```python
from build123d import *

# Parameters (mm, degrees)
F1_DEPTH    = 50.8
F2_R        = 1.75
F3_DEPTH    = 25.4
F5_T4_DEPTH = 50.8
F5_S5_R     = 1.75
F5_T6_DEPTH = 27
F5_S7_R     = 1.75
F5_T8_DEPTH = 27
F2_R_2      = 3
F6_DEPTH    = 7.511
F7_DEPTH    = 2.54
F4_R        = 1.75
F8_DEPTH    = 2.54


# Not quite as in the source:
# - a fillet or chamfer that OpenCascade refuses, or shapes differently, is made with other operations: its cross-section is extruded or revolved along the edge and cut away or added


with BuildPart() as f1:
    # F0 (on Top) → F1 (new body)
    with BuildSketch(Plane.XY):
        Polygon((0, 17.78), (0, 0), (17.78, 0), (17.78, 2.54), (2.54, 2.54), (2.54, 17.78), align=None)
    extrude(amount=F1_DEPTH)

    # F2 (on face) → F3 (cut)
    with BuildSketch(Plane(origin=(0, 0, 0), x_dir=(0, -1, 0), z_dir=(-1, 0, 0))):
        with Locations((-5.65, 9.9)):
            Circle(F2_R)
        with Locations((-5.65, 40.9)):
            Circle(F2_R)
    extrude(amount=-F3_DEPTH, mode=Mode.SUBTRACT)

    # F5: chamfer of 5.08 on 1 edges, made by hand


with BuildPart() as f5_tool2:
    # F5_s3 → F5_t4 (new body)
    with BuildSketch(Plane.XY):
        Polygon((2.54, 7.62), (7.62, 2.54), (2.54, 2.54), align=None)
    extrude(amount=F5_T4_DEPTH)

    # F5_s5 → F5_t6 (cut, symmetric)
    with BuildSketch(Plane.YZ.offset(5.1)):
        with Locations((5.65, 40.9)):
            Circle(F5_S5_R)
    extrude(amount=F5_T6_DEPTH, both=True, mode=Mode.SUBTRACT)

    # F5_s7 → F5_t8 (cut, symmetric)
    with BuildSketch(Plane.YZ.offset(5.1)):
        with Locations((5.65, 9.9)):
            Circle(F5_S7_R)
    extrude(amount=F5_T8_DEPTH, both=True, mode=Mode.SUBTRACT)


with BuildPart() as f1_1:
    add(f1.part)

    # F5_t1: union F5_tool2
    add(f5_tool2.part)

    # F2 (on face) → F6 (cut, through all)
    with BuildSketch(Plane(origin=(0, 0, 0), x_dir=(0, -1, 0), z_dir=(-1, 0, 0))):
        with Locations((-5.65, 40.9)):
            Circle(F2_R_2)
        with Locations((-5.65, 40.9)):
            Circle(F2_R, mode=Mode.SUBTRACT)
        with Locations((-5.65, 9.9)):
            Circle(F2_R_2)
        with Locations((-5.65, 9.9)):
            Circle(F2_R, mode=Mode.SUBTRACT)
    extrude(amount=-F6_DEPTH, mode=Mode.SUBTRACT)

    # F2 (on face) → F7 (join)
    with BuildSketch(Plane(origin=(0, 0, 0), x_dir=(0, -1, 0), z_dir=(-1, 0, 0))):
        with Locations((-5.65, 40.9)):
            Circle(F2_R_2)
        with Locations((-5.65, 40.9)):
            Circle(F2_R, mode=Mode.SUBTRACT)
        with Locations((-5.65, 9.9)):
            Circle(F2_R_2)
        with Locations((-5.65, 9.9)):
            Circle(F2_R, mode=Mode.SUBTRACT)
    extrude(amount=-F7_DEPTH)

    # F4 (on face) → F8 (cut, through all)
    with BuildSketch(Plane.XZ):
        with Locations((12.7, 45.72)):
            Circle(F4_R)
        with Locations((12.7, 5.08)):
            Circle(F4_R)
    extrude(amount=-F8_DEPTH, mode=Mode.SUBTRACT)


solid = f1_1.part
```
CAD build for the part. Positions are in the model's coordinates, mm. A direction names the side the tool comes from. Round coordinates to 2 decimals unless told otherwise and drop trailing zeros. Order: outer loops, then holes, each group sorted by start corner. A loop starts at its lowest first (then second) coordinate and runs counter-clockwise, first axis right, second up. Notation, with made-up numbers: (26.5, -13) - (52.5, -13) arc R22 cw to (52.5, 22) - close; hole circle Ø7 at (76.5, 44). An arc over 180 degrees is marked (long way). Answer in a Markdown table with one row per item. Add a question column.
(1) Mould opens along Z. For faces 4 (the face through (5.6, 4.3, 50.8)), 5 (the face through (1.252, 4.709, 11.376)), 6 (the face through (9, 0, 25)), 7 (the face through (1.252, 3.981, 41.426)) say: +Z half, -Z half, draft (parallel to the pull), parting line (faces both ways), or undercut.
(2) Band-saw the part on B-B on x = 12.7. List the corners of the cut face in (y, z), and give its area (3 significant figures).
(3) 3-axis set-ups, long thin cutter, end or side, ignore diameter. For faces 1 (the face through (10.95, 1.25, 5.16)), 2 (the face through (13, 2.54, 25)), 3 (the face through (4.44, 2.65, 9.8)): which of +Z, -Z, +X, -X, +Y, -Y reach the whole face in a straight line?
(4) Probe L1, parallel to Z at x = 4.2, y = 5.65; L2, parallel to Z at x = 0.85, y = 5.65; L3, parallel to Y at x = 6.25, z = 14.5. List the from-to ranges inside material, lowest first. Write a range as [from, to].
(5) Band-saw the part on D-D on y = 10. List the corners of the cut face in (x, z), and give its area (3 significant figures).
(6) Band-saw the part on C-C on z = 18. List the corners of the cut face in (x, y).
(7) Band-saw the part on A-A on z = 9.9. List the corners of the cut face in (x, y), and give its area (3 significant figures).
(8) Drop flat-ended pins along their axis: pin 1 Ø5 at (y, z) = (14, 27) entering from +X; pin 2 Ø8 at (y, z) = (11, 18.5) entering from +X; pin 3 Ø4 at (y, z) = (5, 20) entering from +X; pin 4 Ø3 at (y, z) = (5.65, 9.9) entering from +X. Give the stop position or say it passes through.
Data:
| question | item | result |
|---|---|---|
| 1 | face 4 | +Z half |
| 1 | face 5 | undercut |
| 1 | face 6 | draft |
| 1 | face 7 | undercut |
| 2 | outline | (0, 0) - (2.54, 0) - (2.54, 3.33) - (0, 3.33) - close; (0, 6.83) - (2.54, 6.83) - (2.54, 43.97) - (0, 43.97) - close; (0, 47.47) - (2.54, 47.47) - (2.54, 50.8) - (0, 50.8) - close |
| 2 | area | 111 mm^2 |
| 3 | face 1 | +Y, -Y |
| 3 | face 2 | +Z, -Z, +X, +Y |
| 3 | face 3 | +X |
| 4 | L1 | z = [0, 6.9], [12.9, 37.9], [43.9, 50.8] |
| 4 | L2 | z = [0, 8.15], [11.65, 39.15], [42.65, 50.8] |
| 4 | L3 | y = [0, 3.91] |
| 5 | outline | (0, 0) - (2.54, 0) - (2.54, 50.8) - (0, 50.8) - close |
| 5 | area | 129 mm^2 |
| 6 | outline | (0, 0) - (17.78, 0) - (17.78, 2.54) - (7.62, 2.54) - (2.54, 7.62) - (2.54, 17.78) - (0, 17.78) - close |
| 7 | outline | (0, 0) - (17.78, 0) - (17.78, 2.54) - (7.62, 2.54) - (7.51, 2.65) - (2.54, 2.65) - (2.54, 3.9) - (0, 3.9) - close; (0, 7.4) - (2.54, 7.4) - (2.54, 17.78) - (0, 17.78) - close |
| 7 | area | 75.5 mm^2 |
| 8 | pin 1 | stops at x = 2.54 |
| 8 | pin 2 | stops at x = 3.16 |
| 8 | pin 3 | stops at x = 7.16 |
| 8 | pin 4 | passes through |
